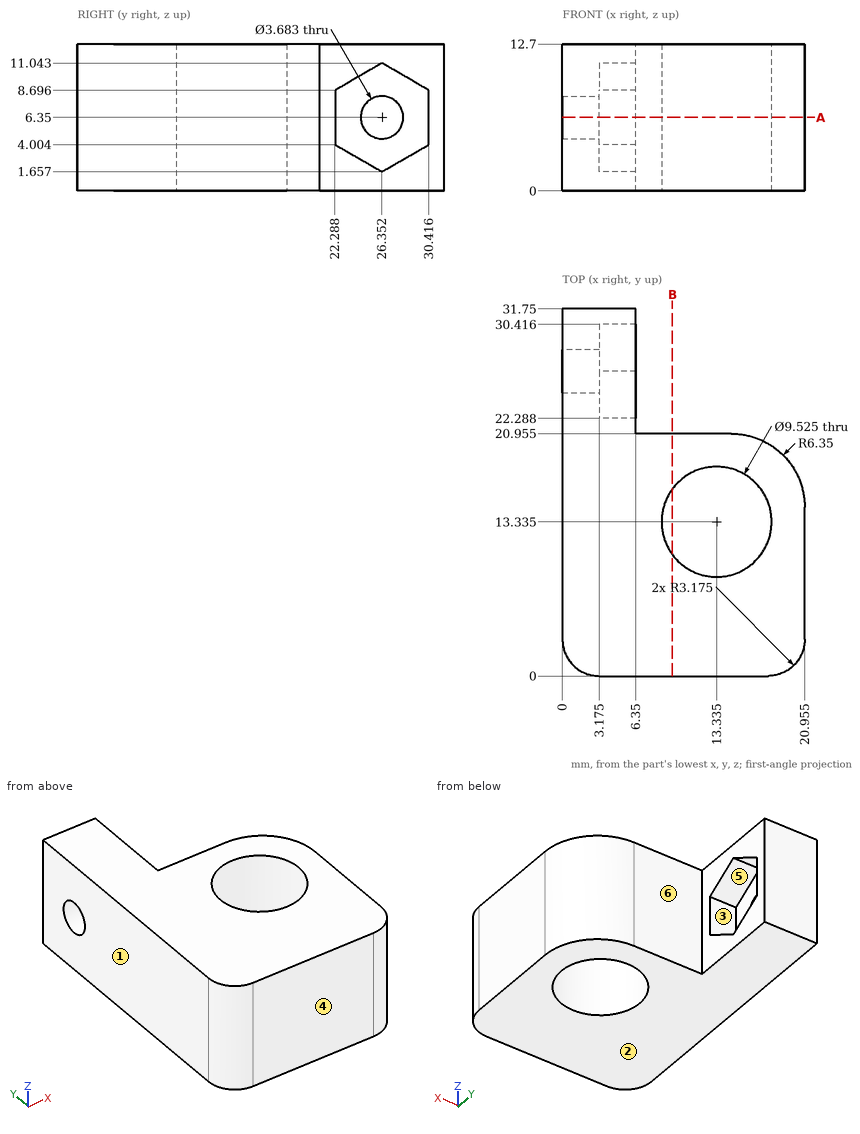
Part print with two shaded views. Sizes in mm from the minimum x, y, z corner. A direction names the side the tool comes from. Coordinates: 2 decimals unless noted, no trailing zeros. Loops run counter-clockwise (first coordinate to the right, second up) from the corner with the lowest first, then second, coordinate; pieces in that order, holes last. Notation, with made-up numbers: M -22,39.5 L -6,39.5 A12 cw -6,49.5 Z; hole C 84.25,33.5 d1. An arc over 180 degrees is marked long. Use CSV: the item, a comma, the result in double quotes. Start each with the question number.
1. Probe probe 1 along Y at (x, z) = (13.5, 12.25) (1 decimal); probe 2 along X at (y, z) = (27, 11); probe 3 along X at (y, z) = (25, 3.75) (1 decimal). List the from-to ranges inside material, lowest first. Write a range as [from, to].
2. Flat gauge pins, fed straight in: pin 1 (3 mm diameter, centred on y = 14, z = 3, fed in from -X); pin 2 (4 mm diameter, centred on x = 9.5, z = 3.5, fed in from +Y) (1 decimal); pin 3 (5 mm diameter, centred on y = 26.35, z = 6.35, fed in from +X) (1 decimal); pin 4 (4 mm diameter, centred on y = 28.5, z = 8, fed in from +X). Where does each tip first touch, or does it go through?
3. Two-plate mould, pull along Z, no slides. Class the marked faces 1, 2 and 3: pulls with the +Z half, pulls with the -Z half, needs draft (parallel to the pull), parting line crosses it, or undercut.
4. Band-saw the part on B-B, the plane x = 9.5. List the corners of the cut face in (y, z) (1 decimal).
5. Band-saw the part on A-A, the plane z = 6.35. Give the number of separate pieces and of enclosed holes in the cut face, then the cut area to 3 significant figures.
6. Tool access for the marked faces 4, 5 and 6: list every direction of +Z, -Z, +X, -X, +Y, -Y with a clear straight run to the whole face (end or side of a thin tool).
Entries:
1,probe 1,"y = [0, 8.6], [18.1, 21]"
1,probe 2,"x = [0, 6.35]"
1,probe 3,"x = [0, 3.2]"
2,pin 1,"stops at x = 0"
2,pin 2,"stops at y = 21"
2,pin 3,"stops at x = 3.2"
2,pin 4,"stops at x = 6.35"
3,face 1,"needs draft"
3,face 2,"pulls with the -Z half"
3,face 3,"undercut"
4,outline,"M 0,0 L 10.5,0 L 10.5,12.7 L 0,12.7 Z; M 16.2,0 L 21,0 L 21,12.7 L 16.2,12.7 Z"
5,separate pieces,"2"
5,enclosed holes,"1"
5,area,"386 mm2"
6,face 4,"+Z, -Z, +X, -X, -Y"
6,face 5,"+X"
6,face 6,"+Z, -Z, +X, +Y"
